Model file for the job. Use its own axes, mm. Face numbers are marked on the shaded views. A direction names the side the tool comes from. Coordinates: 2 decimals unless noted, no trailing zeros. Write each loop counter-clockwise with the first axis right and the second up, starting at its lowest first coordinate (ties: lowest second). Pieces come first, ordered by that corner, then holes. Notation, with made-up numbers: M -2,-7.75 L 52,-7.75 A19 cw 52,18.25 Z; hole C 52.25,50 d11. An arc over 180 degrees is marked long. Put each result on its own line as item: value. Start each with the question number.
Q1. Pull direction Y, two halves, no side cores. Call the marked faces 1, 2 and 3: pulls with the +Y half, pulls with the -Y half, needs draft (parallel to the pull), parting line crosses it, or undercut.
Q2. Cut at D-D (z = 6). Write the cut outline in (x, y), then the cut area to 3 significant figures.
Q3. Cut at C-C (x = 36). Write the cut outline in (y, z).
Q4. Drill centre lines: line 1 along Z through (x, y) = (6.5, 31.75) (3 decimals); line 2 along Z through (x, y) = (4.5, 41.91); line 3 along Z through (x, y) = (43.5, 3). Where is each one in solid material? Low to high.
Q5. Which spindle directions (+Z, -Z, +X, -X, +Y, -Y) get a long thin tool onto all of the face, cutting with end or side? Do the marked faces 4, 5 and 6. Say none if no direction does.
Q6. Drop flat-ended pins along their axis: pin 1 (3 mm diameter, centred on y = 26.5, z = 25, fed in from +X); pin 2 (1 mm diameter, centred on y = 28, z = 7.5, fed in from -X); pin 3 (3 mm diameter, centred on x = 26, z = 28, fed in from +Y); pin 4 (4 mm diameter, centred on x = 22, y = 14.5, fed in from +Z). Give the stop position or say it passes through.
Q7. Cut at B-B (y = 41.91). Write the cut outline in (x, z).
Q8. Cut at A-A (x = 6.5). Write the cut outline in (y, z) (3 decimals), then the cut area to 3 significant figures.
```python
from build123d import *

# Parameters (mm, degrees)
F0_R      = 1.9722998741
F0_R_2    = 4.445
F1_DEPTH  = 10.16
F2_R      = 1.9722998741
F3_DEPTH  = 2.4
F4_R      = 5.08
F5_W      = 50.8
F5_H      = 38.1
F5_R      = 1.9685
F6_DEPTH  = 10.16
F7_R      = 5.08
F8_R      = 1.9685
F9_DEPTH  = 2.4
F11_DEPTH = 10.16
F12_R     = 1.27


# Not quite as in the source:
# - a feature names something its author has since deleted; it is built from what else it names


with BuildPart() as f1:
    # F0 (on Right) → F1 (new body)
    with BuildSketch(Plane.YZ):
        Polygon((15.24, 38.1), (0, 38.1), (0, 0), (31.75, 0), (50.8, 0), (50.8, 50.8), (31.75, 50.8), (21.59, 50.8), (15.24, 50.8), align=None)
        with Locations((21.59, 20.32)):
            Circle(F0_R, mode=Mode.SUBTRACT)
        with BuildLine():
            ThreePointArc((36.195, 20.32), (34.8930896424, 17.1769103576), (31.75, 15.875))
            ThreePointArc((31.75, 15.875), (28.6069103576, 23.4630896424), (36.195, 20.32))
        make_face(mode=Mode.SUBTRACT)
        with Locations((41.91, 20.32)):
            Circle(F0_R, mode=Mode.SUBTRACT)
        with BuildLine():
            ThreePointArc((23.5622998741, 43.688), (20.1953733845, 42.2933733845), (21.59, 45.6602998741))
            ThreePointArc((21.59, 45.6602998741), (22.9846266155, 45.0826266155), (23.5622998741, 43.688))
        make_face(mode=Mode.SUBTRACT)
        with Locations((31.75, 43.688)):
            Circle(F0_R_2, mode=Mode.SUBTRACT)
        with Locations((41.91, 43.688)):
            Circle(F0_R, mode=Mode.SUBTRACT)
    extrude(amount=F1_DEPTH)

    # F2 (on face) → F3 (cut)
    with BuildSketch(Plane.YZ.offset(10.16)):
        Polygon((20.4920916615, 47.0950413284), (18.0904614886, 44.440704152), (19.1883698271, 41.0336628236), (22.6879083385, 40.2809586716), (25.0895385114, 42.935295848), (23.9916301729, 46.3423371764), align=None)
        with Locations((21.59, 43.688)):
            Circle(F2_R, mode=Mode.SUBTRACT)
        Polygon((40.8120916615, 40.2809586716), (44.3116301729, 41.0336628236), (45.4095385114, 44.440704152), (43.0079083385, 47.0950413284), (39.5083698271, 46.3423371764), (38.4104614886, 42.935295848), align=None)
        with Locations((41.91, 43.688)):
            Circle(F2_R, mode=Mode.SUBTRACT)
        Polygon((44.3116301729, 22.9743371764), (40.8120916615, 23.7270413284), (38.4104614886, 21.072704152), (39.5083698271, 17.6656628236), (43.0079083385, 16.9129586716), (45.4095385114, 19.567295848), align=None)
        with Locations((41.91, 20.32)):
            Circle(F2_R, mode=Mode.SUBTRACT)
        Polygon((22.6879083385, 23.7270413284), (19.1883698271, 22.9743371764), (18.0904614886, 19.567295848), (20.4920916615, 16.9129586716), (23.9916301729, 17.6656628236), (25.0895385114, 21.072704152), align=None)
        with Locations((21.59, 20.32)):
            Circle(F2_R, mode=Mode.SUBTRACT)
    extrude(amount=-F3_DEPTH, mode=Mode.SUBTRACT)

    # F4
    f4_edges = [f1.edges().sort_by_distance(p)[0] for p in [
        (5.08, 50.8, 50.8),
        (5.08, 15.24, 50.8),
    ]]
    fillet(f4_edges, radius=F4_R)

    # F5 (on Front) → F6 (join)
    with BuildSketch(Plane.XZ):
        with Locations((25.4, 19.05)):
            Rectangle(F5_W, F5_H)
        with Locations((21.59, 20.32)):
            Circle(F5_R, mode=Mode.SUBTRACT)
        with Locations((41.91, 20.32)):
            Circle(F5_R, mode=Mode.SUBTRACT)
    extrude(amount=-F6_DEPTH)

    # F7
    f7_edges = [f1.edges().sort_by_distance(p)[0] for p in [
        (50.8, 5.08, 38.1),
    ]]
    fillet(f7_edges, radius=F7_R)

    # F8 (on face) → F9 (cut)
    with BuildSketch(Plane(origin=(0, 10.16, 0), x_dir=(-1, 0, 0), z_dir=(0, 1, 0))):
        Polygon((-41.2323596559, 23.8334340491), (-44.613902969, 22.6635707772), (-45.2915433131, 19.1501367281), (-42.5876403441, 16.8065659509), (-39.206097031, 17.9764292228), (-38.5284566869, 21.4898632719), align=None)
        with Locations((-41.91, 20.32)):
            Circle(F8_R, mode=Mode.SUBTRACT)
        Polygon((-24.293902969, 17.9764292228), (-20.9123596559, 16.8065659509), (-18.2084566869, 19.1501367281), (-18.886097031, 22.6635707772), (-22.2676403441, 23.8334340491), (-24.9715433131, 21.4898632719), align=None)
        with Locations((-21.59, 20.32)):
            Circle(F8_R, mode=Mode.SUBTRACT)
    extrude(amount=-F9_DEPTH, mode=Mode.SUBTRACT)

    # F10 (on face) → F11 (join)
    with BuildSketch(Plane(origin=(0, 0, 0), x_dir=(1, 0, 0), z_dir=(0, 0, -1))):
        Polygon((10.16, -10.16), (10.16, -50.8), (50.8, -10.16), align=None)
    extrude(amount=-F11_DEPTH)

    # F12
    f12_edges = [f1.edges().sort_by_distance(p)[0] for p in [
        (10.16, 27.305, 20.32),
        (10.16, 27.305, 43.688),
    ]]
    fillet(f12_edges, radius=F12_R)


solid = f1.part
```
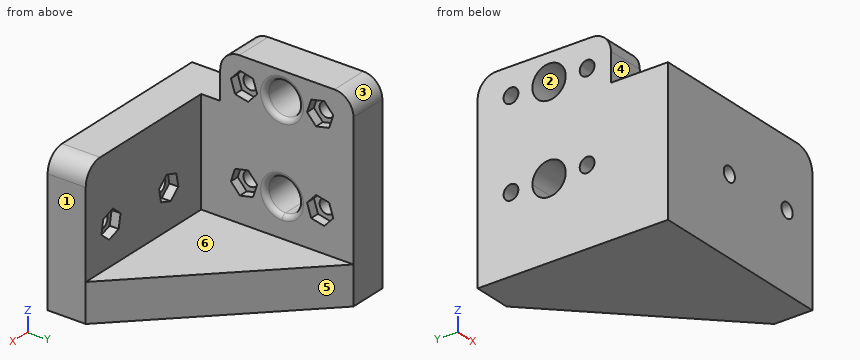
Computed values:
1. face 1: needs draft
1. face 2: undercut
1. face 3: pulls with the +Y half
2. outline: M 0,0 L 50.8,0 L 50.8,10.16 L 10.16,50.8 L 0,50.8 Z
2. area: 1,750 mm2
3. outline: M 0,0 L 24.96,0 L 24.96,10.16 L 10.16,10.16 L 10.16,38.1 L 0,38.1 Z
4. line 1: 0 to 15.875, 24.765 to 39.243, 48.133 to 50.8
4. line 2: 0 to 18.35, 22.29 to 41.72, 45.66 to 50.8
4. line 3: 0 to 19.16, 21.48 to 38.1
5. face 4: +Z, +X, -X, -Y
5. face 5: +Z, -Z, +X, +Y
5. face 6: +Z, +X, +Y
6. pin 1: x = 10.16
6. pin 2: x = 0
6. pin 3: y = 10.16
6. pin 4: z = 10.16
7. outline: M 0,0 L 19.05,0 L 19.05,10.16 L 10.16,10.16 L 10.16,17.15 L 7.76,17.15 L 7.76,18.35 L 0,18.35 Z; M 0,22.29 L 7.76,22.29 L 7.76,23.49 L 10.16,23.49 L 10.16,40.52 L 7.76,40.52 L 7.76,41.72 L 0,41.72 Z; M 0,45.66 L 7.76,45.66 L 7.76,46.86 L 10.16,46.86 L 10.16,50.8 L 0,50.8 Z
8. outline: M 0,0 L 50.8,0 L 50.8,45.72 A5.08 ccw 45.72,50.8 L 20.32,50.8 A5.08 ccw 15.24,45.72 L 15.24,38.1 L 0,38.1 Z; hole C 21.59,20.32 d3.945; hole C 21.59,43.688 d3.945; hole C 31.75,20.32 d8.89; hole C 31.75,43.688 d8.89; hole C 41.91,20.32 d3.945; hole C 41.91,43.688 d3.945
8. area: 2,200 mm2
